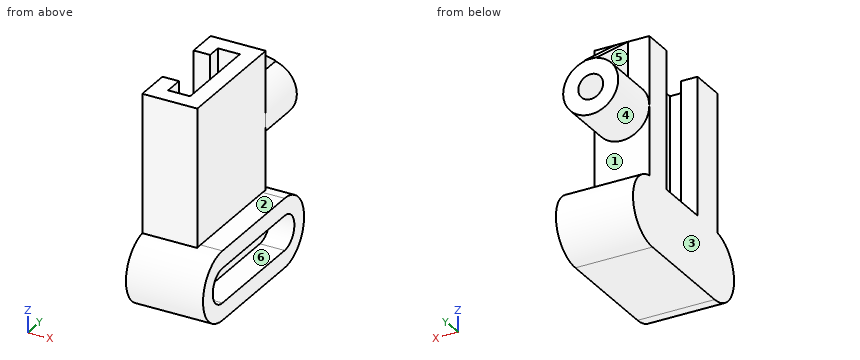
```python
from build123d import *

# Parameters (mm, degrees)
BOSS_EXTRUDE1_DEPTH      = 28
BOSS_EXTRUDE2_DEPTH      = 10
BOSS_EXTRUDE2_DEPTH_BACK = 28
BOSS_EXTRUDE3_DEPTH      = 100
BOSS_EXTRUDE3_DEPTH_BACK = 4
SKETCH4_R                = 20
SKETCH4_R_2              = 9
BOSS_EXTRUDE4_DEPTH      = 40
SKETCH4_2_R              = 9
BOSS_EXTRUDE5_DEPTH      = 8
RIB2_START               = -4.5
RIB2_DEPTH               = 9


with BuildPart() as part:
    # Sketch1 → Boss-Extrude1 (new, symmetric)
    with BuildSketch(Plane(origin=(0, 0, 0), x_dir=(0, 0, -1), z_dir=(1, 0, 0))):
        with BuildLine():
            Line((25, 40), (25, -40))
            ThreePointArc((25, -40), (0, -65), (-25, -40))
            Line((-25, -40), (-25, 40))
            ThreePointArc((-25, 40), (0, 65), (25, 40))
        make_face()
        with BuildLine():
            Line((12.5, 40), (12.5, -40))
            ThreePointArc((12.5, -40), (0, -52.5), (-12.5, -40))
            Line((-12.5, -40), (-12.5, 40))
            ThreePointArc((-12.5, 40), (0, 52.5), (12.5, 40))
        make_face(mode=Mode.SUBTRACT)
    extrude(amount=BOSS_EXTRUDE1_DEPTH, both=True)

    # Sketch1<2> → Boss-Extrude2 (add, two sides: drawn at the far end of the back side and taken through both)
    with BuildSketch(Plane(origin=(0, 0, 0), x_dir=(0, 0, -1), z_dir=(1, 0, 0)).offset(-BOSS_EXTRUDE2_DEPTH_BACK)):
        with BuildLine():
            Line((-12.5, 40), (-12.5, -40))
            ThreePointArc((-12.5, -40), (0, -52.5), (12.5, -40))
            Line((12.5, -40), (12.5, 40))
            ThreePointArc((12.5, 40), (0, 52.5), (-12.5, 40))
        make_face()
    extrude(amount=BOSS_EXTRUDE2_DEPTH + BOSS_EXTRUDE2_DEPTH_BACK)

    # Sketch3 → Boss-Extrude3 (add, two sides: drawn at the far end of the back side and taken through both)
    with BuildSketch(Plane.XY.offset(25).offset(-BOSS_EXTRUDE3_DEPTH_BACK)):
        Polygon((-28, 44), (12, 44), (12, -44), (-28, -44), (-28, -18), (-16, -18), (-16, -32), (0, -32), (0, 32), (-16, 32), (-16, 22), (-28, 22), align=None)
    extrude(amount=BOSS_EXTRUDE3_DEPTH + BOSS_EXTRUDE3_DEPTH_BACK)

    # Sketch4 → Boss-Extrude4 (add)
    with BuildSketch(Plane(origin=(0, 44, 0), x_dir=(1, 0, 0), z_dir=(0, 1, 0))):
        with Locations(Location((-8, -75, 0), (0, 0, 180))):
            Circle(SKETCH4_R)
        with Locations(Location((-8, -75, 0), (0, 0, 270))):
            Circle(SKETCH4_R_2, mode=Mode.SUBTRACT)
    extrude(amount=BOSS_EXTRUDE4_DEPTH)

    # Sketch4<2> → Boss-Extrude5 (add)
    with BuildSketch(Plane(origin=(0, 44, 0), x_dir=(1, 0, 0), z_dir=(0, 1, 0))):
        with Locations(Location((-8, -75, 0), (0, 0, 270))):
            Circle(SKETCH4_2_R)
    extrude(amount=BOSS_EXTRUDE5_DEPTH)

    # Rib2: read off the stored shape, not the designer's step
    # Rib2 outline → Rib2 (add)
    with BuildSketch(Plane.ZY.offset(8).offset(RIB2_START)):
        Polygon((95, 84), (94.48717527, 84), (94.48717527, 44), (125, 44), align=None)
    extrude(amount=RIB2_DEPTH)


solid = part.part
```
Design review of the part built by this model. Coordinates are the model's own, in mm. Face numbers are marked on the shaded views. A direction names the side the tool comes from. Coordinates: 2 decimals unless noted, no trailing zeros. Order: outer loops, then holes, each group sorted by start corner. A loop starts at its lowest first (then second) coordinate and runs counter-clockwise, first axis right, second up. Notation, with made-up numbers: M -27.75,84 L -8.75,84 A4 cw -8.75,88 Z; hole C -18,-7 d3. An arc over 180 degrees is marked long. Answer as a JSON object with one key per item and string values. Group by question number.
1) Add section A-A, the plane x = 22.5. Write out the cut boundary in (y, z), then the cut area to 3 significant figures.
2) Add section D-D, the plane y = -30. Write out the cut boundary in (x, z), then the cut area to 3 significant figures.
3) Wall thickness on L1, parallel to Z at x = 14.5, y = -36.5; L2, parallel to X at y = 66, z = 75; L3, parallel to X at y = -40.5, z = 86: over which ranges is each line inside the solid? List them lowest first.
4) Add section C-C, the plane z = 38.5. Write out the cut boundary in (x, y), then the cut area to 3 significant figures.
5) For pin 1 (5 mm diameter, centred on x = -18.5, z = 74.5, fed in from -Y); pin 2 (12.5 mm diameter, centred on y = -9, z = 5, fed in from +X); pin 3 (13 mm diameter, centred on x = 22, y = -2, fed in from +Z); pin 4 (9 mm diameter, centred on y = 71, z = 112.5, fed in from -X), all flat-tipped, find the tip position at first contact; note any pin that passes through.
6) Mouldability with a two-part tool opening along Z and no side actions: class the marked faces 1, 2 and 3 as pulls with the +Z half, pulls with the -Z half, needs draft (parallel to the pull), parting line crosses it, or undercut.
7) Add section B-B, the plane y = 73. Write out the cut boundary in (x, z).
8) Tool access review of the marked faces 4, 5 and 6: name each direction out of +Z, -Z, +X, -X, +Y, -Y from which nothing blocks a thin tool from reaching the whole face with its end or side.
Computed values:
{
 "1": {"outline": "M -40,-25 L 40,-25 A25 ccw 40,25 L -40,25 A25 ccw Z; hole M -40,-12.5 L 40,-12.5 A12.5 ccw 40,12.5 L -40,12.5 A12.5 ccw Z", "area": "3,470 mm^2"},
 "2": {"outline": "M -28,-25 L 28,-25 L 28,-12.5 L 10,-12.5 L 10,12.5 L 28,12.5 L 28,25 L 12,25 L 12,125 L 0,125 L 0,25 L -16,25 L -16,125 L -28,125 Z", "area": "4,750 mm^2"},
 "3": {"L1": "z = -25 to -12.5, 12.5 to 25", "L2": "x = -28 to -17, 1 to 12", "L3": "x = -28 to 12"},
 "4": {"outline": "M -28,-44 L 12,-44 L 12,44 L -28,44 L -28,22 L -16,22 L -16,32 L 0,32 L 0,-32 L -16,-32 L -16,-18 L -28,-18 Z", "area": "2,020 mm^2"},
 "5": {"pin 1": "stops at y = -44", "pin 2": "stops at x = 10", "pin 3": "stops at z = 25", "pin 4": "passes through"},
 "6": {"face 1": "undercut", "face 2": "pulls with the +Z half", "face 3": "needs draft"},
 "7": {"outline": "M -12.5,94.49 A20 ccw long -3.5,94.49 L -3.5,103.25 L -12.5,103.25 Z; hole C -8,75 d18"},
 "8": {"face 4": "+Y", "face 5": "+Z, -X, +Y", "face 6": "+X"}
}
